Can you work these out from the model? Positions are in its coordinate system, mm. A direction names the side the tool comes from. Coordinates: 2 decimals unless noted, no trailing zeros. Order: outer loops, then holes, each group sorted by start corner. A loop starts at its lowest first (then second) coordinate and runs counter-clockwise, first axis right, second up. Notation, with made-up numbers: (54.5, 67) - (93.5, 67) arc R8 cw to (93.5, 76) - close; hole circle Ø9 at (-15.75, 7). An arc over 180 degrees is marked (long way). Return JSON: item names as keys, results as strings. Group by question number.
1) Imagine slicing it at D-D (x = 80.5). Write out the boundary of the cut face in (y, z), and give its area (3 significant figures).
2) If I drill on line 1 along X through (y, z) = (2.25, -3); line 2 along Z through (x, y) = (16, 0.25), over which ranges is the centre line in solid material (lowest first)?
3) Which directions (+Z, -Z, +X, -X, +Y, -Y) give clear straight access to the entire face, cutting with the end or side of a thin tool? Please do faces 1 (the face through (94, 0, 0)), 2 (the face through (3.29, -0.54, 2.44)), 3 (the face through (86, 0, 2)).
4) Imagine slicing it at A-A (y = 0). Write out the boundary of the cut face in (x, z), and give its area (4 significant figures).
5) For pin 1 Ø5 at (y, z) = (-4, 3.5) entering from -X; pin 2 Ø5 at (x, y) = (25.5, -3) entering from -Z, each with a flat end and sliding along its axis, tell me the tip position at first contact or that it passes through.
6) Imagine slicing it at C-C (x = 61.5). Write out the boundary of the cut face in (y, z).
```python
from build123d import *

# Parameters (mm, degrees)
CHAMFER1_SIZE = 0.5


with BuildPart() as part:
    # Sketch1 → Revolve1 (revolve)
    with BuildSketch(Plane.XY):
        Polygon((0, 0), (0, 2.5), (6, 2.5), (6, 5), (74, 5), (74, 2.5), (79, 2.5), (79, 2), (94, 2), (94, 0), align=None)
    revolve(axis=Axis((94, 0, 0), (-1, 0, 0)))

    # Chamfer1
    chamfer1_edges = [part.edges().sort_by_distance(p)[0] for p in [
        (0, -2.5, 0),
        (94, -2, 0),
    ]]
    chamfer(chamfer1_edges, length=CHAMFER1_SIZE)


solid = part.part
```
Calculated:
{
 "1": {"outline": "circle Ø4 at (0, 0)", "area": "12.6 mm2"},
 "2": {"line 1": "6 to 74", "line 2": "-4.99 to 4.99"},
 "3": {"face 1": "+Z, -Z, +X, +Y, -Y", "face 2": "-X", "face 3": "+X"},
 "4": {"outline": "(0, -2) - (0.5, -2.5) - (6, -2.5) - (6, -5) - (74, -5) - (74, -2.5) - (79, -2.5) - (79, -2) - (93.5, -2) - (94, -1.5) - (94, 1.5) - (93.5, 2) - (79, 2) - (79, 2.5) - (74, 2.5) - (74, 5) - (6, 5) - (6, 2.5) - (0.5, 2.5) - (0, 2) - close", "area": "794.5 mm2"},
 "5": {"pin 1": "x = 6", "pin 2": "z = -4.97"},
 "6": {"outline": "circle Ø10 at (0, 0)"}
}
